Part model, mm, in its own coordinate system. A direction names the side the tool comes from. Give positions to 0.01 mm unless a question says otherwise; leave off trailing zeros. Loops run counter-clockwise (first coordinate to the right, second up) from the corner with the lowest first, then second, coordinate; pieces in that order, holes last. Notation, with made-up numbers: M -8,-39 L -1,-39 A20 ccw -1,-12 Z; hole C -14,54.25 d10. An arc over 180 degrees is marked long. Answer in a Markdown table with one row per item.
Autodesk Inventor part; units mm, degrees
ref_plane "YZ Plane" through (0, 0, 0) normal (1, 0, 0) x (0, 1, 0)
ref_plane "XZ Plane" through (0, 0, 0) normal (0, 1, 0) x (-1, 0, 0)
ref_plane "XY Plane" through (0, 0, 0) normal (0, 0, 1) x (1, 0, 0)
sketch "Sketch1" plane through (0, 0, 0) normal (0, 0, 1) x (1, 0, 0)
  circle A0 centre (0, 0) radius 39.25
  circle A1 centre (0, 0) radius 42.5
  line L0 (39.2468, 0.5) -> (42.4971, 0.5)
  line L1 (44.2943, 0.5) -> (44.2943, -0.5)
  line L2 (42.497, -0.5013) -> (39.2468, -0.5013)
  line L3 (38.2943, -0.5) -> (38.2943, 0.5)
  line L4 (-6, 42.55) -> (6, 42.55)
  line L5 (6, 42.55) -> (6, 38.73)
  line L6 (6, 38.73) -> (-6, 38.73)
  line L7 (-6, 38.73) -> (-6, 42.55)
  point P0 (-6, 42.0743)
  point P1 (6, 42.0743)
  dimension "d0" = 78.5
  dimension "d1" = 85
  dimension "d2" = 6
  dimension "d3" = 1
  dimension "d4" = 0.5
  dimension "d7" = 12
  dimension "d8" = 6
  dimension "d9" = 42.55
extrude "Extrusion1" add sketch "Sketch1" along normal blind 75 contours A0 L5 A1 L0 | L2 A1 L7 A0 | A0 L7 A1 L5 | A1 L7 L4 L5
sketch "Sketch3" plane through (39.2468, 0.5, 0) normal (0, -1, 0) x (1, 0, 0)
  line L0 (3.2502, 0) -> (-33.2468, 0)
  line L1 (2.9121, 0) -> (9.9121, 0)
  line L2 (12.9121, 3) -> (12.9121, 12)
  line L3 (9.9121, 15) -> (2.9121, 15)
  line L4 (2.9121, 15) -> (2.9121, 0)
  arc A0 (12.9121, 12) -> (9.9121, 15) centre (9.9121, 12) ccw
  arc A1 (9.9121, 0) -> (12.9121, 3) centre (9.9121, 3) ccw
  point P0 (-39.2468, 0)
  point P1 (12.9121, 15)
  point P2 (12.9121, 0)
  dimension "d10" = 10
  dimension "d11" = 15
  dimension "d12" = 3
extrude "Extrusion2" add sketch "Sketch3" against normal blind 4
sketch "Sketch4" plane through (39.2468, 4.5, 0) normal (0, 1, 0) x (1, 0, 0)
  circle A0 centre (7.8143, -7.5) radius 3.5
  line L0 (9.9121, 0) -> (3.0143, 0)
  line L1 (3.0143, -15) -> (3.0143, 0)
  point P0 (-39.2468, 0)
  point P1 (3.0143, -7.5)
  dimension "d15" = 7
  dimension "d16" = 7.5
  dimension "d17" = 4.8
extrude "Extrusion3" cut sketch "Sketch4" against normal blind 1.5
sketch "Sketch5" plane through (47.0611, 3, 7.5) normal (0, 1, 0) x (1, 0, 0)
  circle A0 centre (0, 0) radius 3.5
  point P0 (-47.0611, 7.5)
hole "Hole1" at (47.0611, 3, 7.5) direction (0, -1, 0) diameter 3.2 end through all
mirror "Mirror1" about plane through (0, 0, 0) normal (0, 1, 0) of "Extrusion2", "Extrusion3", "Hole1"
sketch "Sketch6" plane through (-6, 42.55, 0) normal (0, 1, 0) x (1, 0, 0)
  line L0 (0, 0) -> (0, -75)
  line L1 (12, 0) -> (12, -75)
  line L2 (0, -13) -> (12, -13)
  line L3 (12, -13) -> (12, -39)
  line L4 (12, -39) -> (0, -39)
  line L5 (0, -39) -> (0, -13)
  circle A0 centre (9.5, -15.75) radius 1.35
  circle A1 centre (9.5, -36.25) radius 1.35
  line L6 (12, 0) -> (0, 0)
  line L7 (2.9, -72) -> (9.1, -72)
  line L8 (9.1, -72) -> (9.1, -46)
  line L9 (9.1, -46) -> (2.9, -46)
  line L10 (2.9, -46) -> (2.9, -72)
  line L11 (12, -75) -> (0, -75)
  circle A2 centre (6, -69.5) radius 1.35
  circle A3 centre (6, -48.5) radius 1.35
  line L12 (2.9, -51.7) -> (9.1, -51.7)
  line L13 (9.1, -51.7) -> (9.1, -66.3)
  line L14 (9.1, -66.3) -> (2.9, -66.3)
  line L15 (2.9, -66.3) -> (2.9, -51.7)
  point P0 (6, 0)
  point P1 (6, -46)
  point P2 (2.9, -66.3)
  point P3 (9.1, -51.7)
  dimension "d27" = 26
  dimension "d28" = 2.7
  dimension "d29" = 2.7
  dimension "d30" = 2.75
  dimension "d31" = 2.5
  dimension "d32" = 2.5
  dimension "d33" = 2.75
  dimension "d34" = 13
  dimension "d35" = 6.2
  dimension "d36" = 26
  dimension "d37" = 2.9
  dimension "d38" = 3
  dimension "d39" = 2.7
  dimension "d40" = 2.7
  dimension "d41" = 2.5
  dimension "d42" = 2.5
  dimension "d43" = 3.1
  dimension "d44" = 3.1
  dimension "d47" = 14.6
  dimension "d48" = 5.7
extrude "Extrusion4" cut sketch "Sketch6" against normal blind 6 contours A0 | A1 | L10 L12 L8 L14 | A2 | A3
chamfer "Chamfer1" distance 1 angle 45 1 edges at (-39.25, 0.0006, 0)
equation "\"d29\" = d28"
equation "\"d32\" = d31"
equation "\"d33\" = d30"
equation "\"d40\" = d39"
equation "\"d44\" = d43"
properties part number "sensor_adapter"
(1) Saw through at B-B (z = 7.5). Give the number of separate pieces and of enclosed holes in the cut face, plus the area to 3 significant figures.
Recorded:
| item | result |
|---|---|
| separate pieces | 3 |
| enclosed holes | 0 |
| area | 875 mm^2 |
(2) Saw through at D-D (z = 39.5). Write the cut outline in (x, y), plus the area to 3 significant figures.
Recorded:
| item | result |
|---|---|
| outline | M -6,42.07 A42.5 ccw long 42.5,-0.5 L 39.25,-0.5 A39.25 cw long 39.25,0.5 L 42.5,0.5 A42.5 ccw 6,42.07 L 6,42.55 L -6,42.55 Z |
| area | 834 mm^2 |
(3) Drill centre lines: line 1 along Z through (x, y) = (3.5, 41.4); line 2 along Z through (x, y) = (0, 41); line 3 along X through (y, z) = (2.2, 7.5). Where is each one in solid material? Low to high.
Recorded:
| item | result |
|---|---|
| line 1 | z = 0 to 14.4, 17.1 to 34.9, 37.6 to 75 |
| line 2 | z = 0 to 47.15, 49.85 to 51.7, 66.3 to 68.15, 70.85 to 75 |
| line 3 | x = -42.44 to -39.19, 39.19 to 45.46, 48.66 to 52.16 |
(4) Pull direction Y, two halves, no side cores. Call faces 4 (the face through (31.659, 28.354, 36.975)), 5 (the face through (41, 0.5, 20)), 6 (the face through (-0.29, 40.91, 49.82)): +Y half, -Y half, draft (parallel to the pull), parting line (faces both ways), or undercut.
Recorded:
| item | result |
|---|---|
| face 4 | +Y half |
| face 5 | undercut |
| face 6 | draft |
(5) Saw through at A-A (x = 0). Write the cut outline in (y, z).
Recorded:
| item | result |
|---|---|
| outline | M -42.5,0 L -40.25,0 L -39.25,1 L -39.25,75 L -42.5,75 Z; M 39.25,1 L 40.25,0 L 42.55,0 L 42.55,47.15 L 39.25,47.15 Z; M 39.25,49.85 L 42.55,49.85 L 42.55,51.7 L 39.25,51.7 Z; M 39.25,66.3 L 42.55,66.3 L 42.55,68.15 L 39.25,68.15 Z; M 39.25,70.85 L 42.55,70.85 L 42.55,75 L 39.25,75 Z |
(6) Pin check, flat tips, straight feed: pin 1 Ø2 at (x, z) = (0, 48.5) entering from +Y; pin 2 Ø4 at (x, z) = (47.06, 7.5) entering from -Y; pin 3 Ø12 at (y, z) = (28, 64) entering from +X. Stop position of each tip, or through.
Recorded:
| item | result |
|---|---|
| pin 1 | stops at y = -39.24 |
| pin 2 | stops at y = -3 |
| pin 3 | stops at x = 36.36 |
(7) Which spindle directions (+Z, -Z, +X, -X, +Y, -Y) get a long thin tool onto all of the face, cutting with end or side? Do faces 1 (the face through (49, 3, 8)), 2 (the face through (51.3, 2.5, 14.1)), 3 (the face through (47.2, -0.5, 9.3)). Say none if no direction does.
Recorded:
| item | result |
|---|---|
| face 1 | +Y |
| face 2 | +Z, +X, +Y, -Y |
| face 3 | +Z, -Z, +X |
(8) Saw through at C-C (z = 69.5). Write the cut outline in (x, y).
Recorded:
| item | result |
|---|---|
| outline | M -6,42.07 A42.5 ccw long 42.5,-0.5 L 39.25,-0.5 A39.25 cw long -1.35,39.23 L -1.35,42.55 L -6,42.55 Z; M 1.35,39.23 A39.25 cw 39.25,0.5 L 42.5,0.5 A42.5 ccw 6,42.07 L 6,42.55 L 1.35,42.55 Z |
